For this review, use the dimensioned drawing (mm, ordinates from the lowest corner) and the shaded views. A direction names the side the tool comes from. Round coordinates to 2 decimals unless told otherwise and drop trailing zeros. Loops run counter-clockwise (first coordinate to the right, second up) from the corner with the lowest first, then second, coordinate; pieces in that order, holes last. Notation, with made-up numbers: M 27.5,-2.5 L 55.5,-2.5 A19 ccw 55.5,4.5 Z; hole C 68,85.25 d9. An arc over 180 degrees is marked long. One line per item, written item: value. Start each with the question number.
Item 1: Mouldability with a two-part tool opening along X and no side actions: class the marked faces 1, 2, 3 and 4 as released by +X, released by -X, zero draft, split by the parting line, or undercut.
Item 2: We need section B-B (x = 29.1). Write out the cut boundary in (y, z), then the cut area to 3 significant figures.
Item 3: For line 1 along X through (y, z) = (1.5, 6); line 2 along X through (y, z) = (0.9, 9.5); line 3 along Z through (x, y) = (14.5, 0.1), list the stretches that pass through material, from the lowest coordinate up.
Item 4: For the marked faces 5 and 6, list the 3-axis set-ups (+Z, -Z, +X, -X, +Y, -Y) from which the entire face can be reached by the end or side of a thin tool; tool diameter is ignored.
Item 5: We need section C-C (y = 1.1). Write out the cut boundary in (x, z), then the cut area to 3 significant figures.
Item 6: We need section D-D (z = 2.5). Write out the cut boundary in (x, y).
Item 7: Clearance check with a flat-ended pin moving along its axis: pin 1 (4 mm diameter, centred on x = 18.5, z = 10, fed in from +Y). State where the tip first meets the part, or that it passes through.
Item 8: We need section A-A (z = 6). Write out the cut boundary in (x, y).
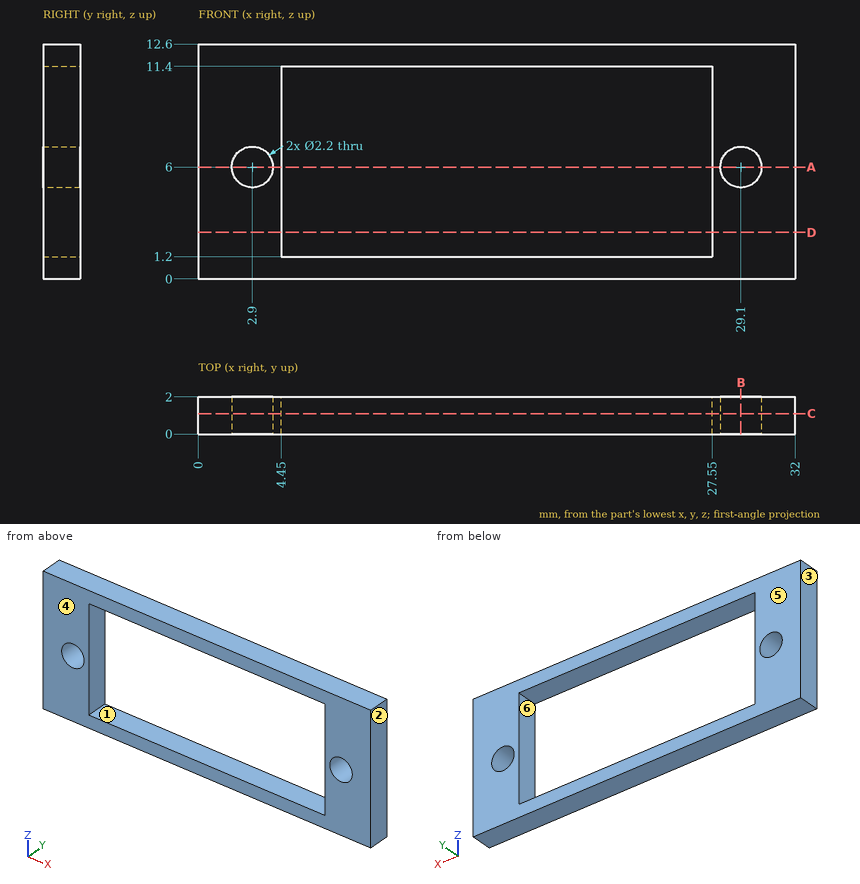
A:
1. face 1: undercut
1. face 2: released by +X
1. face 3: released by -X
1. face 4: zero draft
2. outline: M 0,0 L 2,0 L 2,4.9 L 0,4.9 Z; M 0,7.1 L 2,7.1 L 2,12.6 L 0,12.6 Z
2. area: 20.8 mm2
3. line 1: 0 to 1.8, 4 to 4.45, 27.55 to 28, 30.2 to 32
3. line 2: 0 to 4.45, 27.55 to 32
3. line 3: 0 to 1.2, 11.4 to 12.6
4. face 5: +Z, -Z, +X, -X, +Y
4. face 6: +Y, -Y
5. outline: M 0,0 L 32,0 L 32,12.6 L 0,12.6 Z; hole C 2.9,6 d2.2; hole M 4.45,1.2 L 27.55,1.2 L 27.55,11.4 L 4.45,11.4 Z; hole C 29.1,6 d2.2
5. area: 160 mm2
6. outline: M 0,0 L 4.45,0 L 4.45,2 L 0,2 Z; M 27.55,0 L 32,0 L 32,2 L 27.55,2 Z
7. pin 1: y = 2
8. outline: M 0,0 L 1.8,0 L 1.8,2 L 0,2 Z; M 4,0 L 4.45,0 L 4.45,2 L 4,2 Z; M 27.55,0 L 28,0 L 28,2 L 27.55,2 Z; M 30.2,0 L 32,0 L 32,2 L 30.2,2 Z
